For this review, take the finished solid that the model builds, in its own axes (mm). Coordinates: 2 decimals unless noted, no trailing zeros. Order: outer loops, then holes, each group sorted by start corner. A loop starts at its lowest first (then second) coordinate and runs counter-clockwise, first axis right, second up.
from build123d import *

# Parameters (mm, degrees)
F0_W     = 19.05
F0_H     = 76.2
F1_DEPTH = 939.8
F2_W     = 88.9
F2_H     = 38.1
F3_DEPTH = 609.6
F4_SIZE  = 19.05
F5_W     = 19.05
F5_H     = 76.2
F6_DEPTH = 939.8
F7_R     = 12.7


with BuildPart() as f1:
    # F0 (on Right) → F1 (new body, symmetric)
    with BuildSketch(Plane.YZ):
        with Locations((-9.525, 571.5)):
            Rectangle(F0_W, F0_H)
    extrude(amount=F1_DEPTH, both=True)

    # F2 (on face) → F3 (join, through all)
    with BuildSketch(Plane.XY.offset(609.6)):
        with Locations((590.55, -19.05)):
            Rectangle(F2_W, F2_H)
        with Locations((-590.55, -19.05)):
            Rectangle(F2_W, F2_H)
    extrude(amount=-F3_DEPTH)

    # F4
    f4_edges = [f1.edges().sort_by_distance(p)[0] for p in [
        (590.55, -38.1, 0),
        (-590.55, -38.1, 0),
    ]]
    chamfer(f4_edges, length=F4_SIZE)

    # F5 (on Right) → F6 (join, symmetric)
    with BuildSketch(Plane.YZ):
        with Locations((-9.525, 393.7)):
            Rectangle(F5_W, F5_H)
    extrude(amount=F6_DEPTH, both=True)

    # F7
    f7_edges = [f1.edges().sort_by_distance(p)[0] for p in [
        (939.8, -9.525, 609.6),
        (939.8, -9.525, 533.4),
        (590.55, -38.1, 609.6),
        (635, -28.575, 609.6),
        (546.1, -28.575, 609.6),
        (635, -38.1, 314.325),
        (546.1, -38.1, 314.325),
        (-590.55, -38.1, 609.6),
        (-546.1, -38.1, 314.325),
        (-635, -38.1, 314.325),
        (-635, -28.575, 609.6),
        (-939.8, -9.525, 609.6),
        (-939.8, -9.525, 533.4),
        (-546.1, -28.575, 609.6),
        (-590.55, -38.1, 19.05),
        (590.55, -38.1, 19.05),
        (939.8, -9.525, 431.8),
        (939.8, -9.525, 355.6),
        (-939.8, -9.525, 431.8),
        (-939.8, -9.525, 355.6),
    ]]
    fillet(f7_edges, radius=F7_R)


solid = f1.part
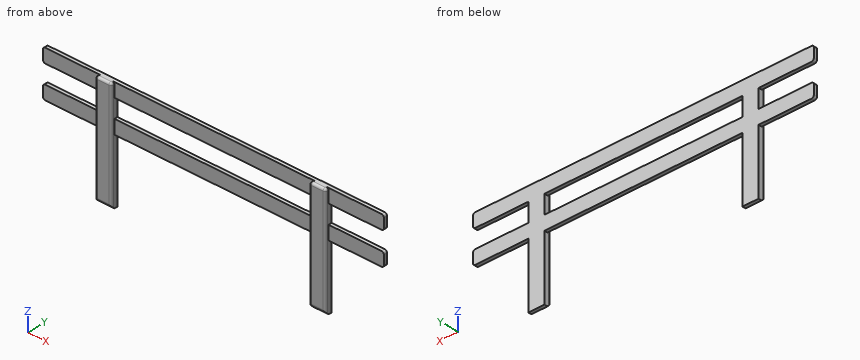
1. Take a section at A-A, the plane x = 245. Give the boundary of the cut face in (y, z).
Answer below:
outline: (-19.05, 355.6) - (0, 355.6) - (0, 431.8) - (-19.05, 431.8) - close; (-19.05, 533.4) - (0, 533.4) - (0, 609.6) - (-19.05, 609.6) - close
2. Clearance check with flat-ended pins moving along their axes: pin 1 Ø2 at (y, z) = (-18, 107.5) entering from -X; pin 2 Ø23 at (x, z) = (-799.5, 397.5) entering from -Y; pin 3 Ø21 at (x, y) = (-203, -9.5) entering from -Z. State where each tip first meets the part, or that it passes through.
Answer below:
pin 1: stops at x = -635
pin 2: stops at y = -19.05
pin 3: stops at z = 355.6
3. To check wall thickness, follow L1, parallel to X at y = -1.5, z = 258.5; L2, parallel to X at y = -28, z = 100.5; L3, parallel to Z at x = -827, y = -4. State the ranges of each line that lie inside material, in increasing order.
Answer below:
L1: x = -635 to -546.1, 546.1 to 635
L2: x = -634.73 to -546.37, 546.37 to 634.73
L3: z = 355.6 to 431.8, 533.4 to 609.6
4. Take a section at B-B, the plane z = 149. Give the boundary of the cut face in (x, y).
Answer below:
outline: (-635, -25.4) arc R12.7 ccw to (-622.3, -38.1) - (-558.8, -38.1) arc R12.7 ccw to (-546.1, -25.4) - (-546.1, 0) - (-635, 0) - close; (546.1, -25.4) arc R12.7 ccw to (558.8, -38.1) - (622.3, -38.1) arc R12.7 ccw to (635, -25.4) - (635, 0) - (546.1, 0) - close
